Design review of the part shown in the three views and the two pictorial views. Dimensions are in mm from the part's minimum x, y and z. Give positions to 0.01 mm unless a question says otherwise; leave off trailing zeros. Write each loop counter-clockwise with the first axis right and the second up, starting at its lowest first coordinate (ties: lowest second). Pieces come first, ordered by that corner, then holes. Notation, with made-up numbers: M 75.25,34.5 L 86.25,34.5 A17 ccw 86.25,42.5 Z; hole C -40,27.5 d8. An arc over 180 degrees is marked long. Use one line per item in the form item = value. Start each with the question number.
Q1. Clearance check with flat-ended pins moving along their axes: pin 1 Ø2 at (x, y) = (79, 31) entering from +Z; pin 2 Ø18.5 at (x, y) = (44.5, 50) entering from +Z; pin 3 Ø12 at (y, z) = (31.5, 9) entering from -X; pin 4 Ø2 at (y, z) = (57, 19) entering from +X. State where each tip first meets the part, or that it passes through.
Q2. Consider section A-A on y = 50. Write out the cut boundary in (x, z), and give its area (3 significant figures).
Q3. Consider section B-B on x = 44.5. Write out the cut boundary in (y, z), and give its area (3 significant figures).
Q4. Consider section D-D on y = 75. Write out the cut boundary in (x, z), and give its area (3 significant figures).
Q5. Consider section C-C on z = 13. Write out the cut boundary in (x, y), and give its area (3 significant figures).
Q6. For probe 1 along Y at (x, z) = (44, 35); probe 2 along X at (y, z) = (48.5, 16.5); probe 3 along Z at (x, y) = (36.5, 59), list the stretches that pass through material, from the lowest coordinate up. Write a range as [from, to].
Q7. Mouldability with a two-part tool opening along X and no side actions: class the marked faces 1, 2 and 3 as released by +X, released by -X, zero draft, split by the parting line, or undercut.
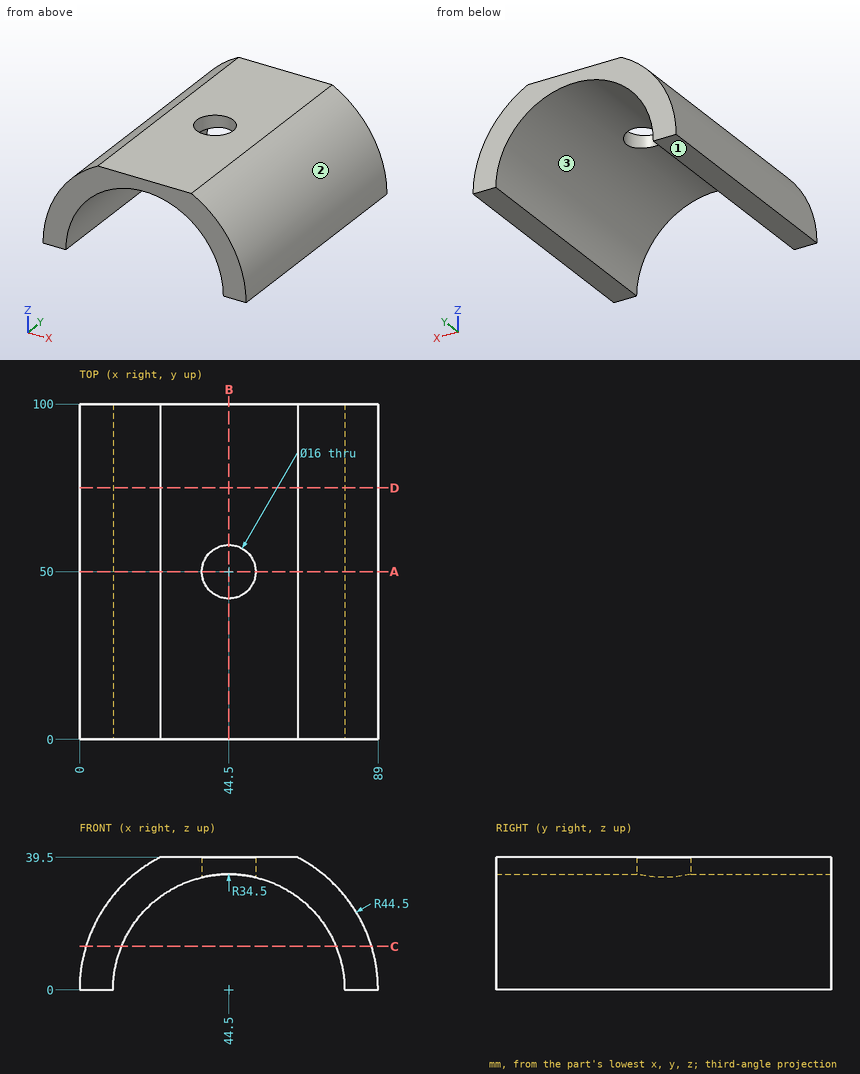
Working result:
q1.pin_1 = 29.29
q1.pin_2 = 39.5
q1.pin_3 = 0.1
q1.pin_4 = 85.2
q2.outline = M 0,0 L 10,0 A34.5 cw 36.5,33.56 L 36.5,39.5 L 24.01,39.5 A44.5 ccw Z; M 52.5,33.56 A34.5 cw 79,0 L 89,0 A44.5 ccw 64.99,39.5 L 52.5,39.5 Z
q2.area = 1,020 mm²
q3.outline = M 0,34.5 L 42,34.5 L 42,39.5 L 0,39.5 Z; M 58,34.5 L 100,34.5 L 100,39.5 L 58,39.5 Z
q3.area = 420 mm²
q4.outline = M 0,0 L 10,0 A34.5 cw 79,0 L 89,0 A44.5 ccw 64.99,39.5 L 24.01,39.5 A44.5 ccw Z
q4.area = 1,100 mm²
q5.outline = M 1.94,0 L 12.54,0 L 12.54,100 L 1.94,100 Z; M 76.46,0 L 87.06,0 L 87.06,100 L 76.46,100 Z
q5.area = 2,120 mm²
q6.probe_1 = [0, 42.02], [57.98, 100]
q6.probe_2 = [3.17, 14.2], [74.8, 85.83]
q6.probe_3 = [33.56, 39.5]
q7.face_1 = zero draft
q7.face_2 = released by +X
q7.face_3 = undercut
